```python
from build123d import *

# Parameters (mm, degrees)
F1_DEPTH = 76.2
F2_R     = 7.702083685
F3_DEPTH = 76.2


# Not quite as in the source:
# - a feature names something its author has since deleted; it is built from what else it names


with BuildPart() as f1:
    # F0 (on Front) → F1 (new body)
    with BuildSketch(Plane.XZ):
        Polygon((-37.524404479, 59.8273601898), (-37.524404479, -16.3726398102), (38.675595521, -16.3726398102), (38.675595521, 59.8273601898), (35.8841840983, 59.8273601898), align=None)
    extrude(amount=F1_DEPTH)

    # F2 (on face) → F3 (cut)
    with BuildSketch(Plane.XZ.offset(76.2)):
        with Locations((-8.9478027076, 33.3981923759)):
            Circle(F2_R)
    extrude(amount=-F3_DEPTH, mode=Mode.SUBTRACT)


solid = f1.part
```
Geometry check sheet. Reference: the model listing, model coordinates, mm. Coordinates: 2 decimals unless noted, no trailing zeros. Order: outer loops, then holes, each group sorted by start corner. A loop starts at its lowest first (then second) coordinate and runs counter-clockwise, first axis right, second up. Notation, with made-up numbers: M 22.25,89 L 29.25,89 A15 ccw 29.25,110 Z; hole C -21.75,61 d10. An arc over 180 degrees is marked long. One line per question, with ' | ' between items. Start each with the question number.
Item 1: Draft check along X on faces 1 (the flat face through (-37.524, -38, 22)), 2 (the flat face through (38.676, -38, 21)), 3 (the cylindrical face through (-10.62, -38.63, 25.88)), 4 (the flat face through (0, -38, -16.373)). Enter one of: pulls with the +X half, pulls with the -X half, needs draft (parallel to the pull), parting line crosses it, or undercut.
Item 2: Cross-section at B-B on x = -15.5. Enter the section's corners in (y, z), then the cut area to 3 significant figures.
Item 3: Cross-section at A-A on z = 37.5. Enter the section's corners in (x, y).
Item 4: Material ranges on L1, parallel to Z at x = -3.5, y = -34; L2, parallel to X at y = -50, z = 40; L3, parallel to Z at x = -7.5, y = -42, recorded low to high. Write a range as [from, to].
Item 5: Gauge pin test, flat end, axial feed: pin 1 (20 mm diameter, centred on x = -8.95, z = 33.4, fed in from +Y). Record the tip position at first contact, or that the pin passes through.
Item 6: Cross-section at C-C on y = -31. Enter the section's corners in (x, z), then the cut area to 3 significant figures.
Findings:
1) face 1: pulls with the -X half | face 2: pulls with the +X half | face 3: undercut | face 4: needs draft
2) outline: M -76.2,-16.37 L 0,-16.37 L 0,29.35 L -76.2,29.35 Z; M -76.2,37.45 L 0,37.45 L 0,59.83 L -76.2,59.83 Z | area: 5,190 mm²
3) outline: M -37.52,-76.2 L -15.47,-76.2 L -15.47,0 L -37.52,0 Z; M -2.43,-76.2 L 38.68,-76.2 L 38.68,0 L -2.43,0 Z
4) L1: z = [-16.37, 27.95], [38.84, 59.83] | L2: x = [-37.52, -12.91], [-4.98, 38.68] | L3: z = [-16.37, 25.83], [40.96, 59.83]
5) pin 1: stops at y = 0
6) outline: M -37.52,-16.37 L 38.68,-16.37 L 38.68,59.83 L -37.52,59.83 Z; hole C -8.95,33.4 d15.4 | area: 5,620 mm²
